Read the model definition and answer for the solid it produces. Units are mm, in the model's axes. Face numbers are marked on the shaded views. A direction names the side the tool comes from. Give positions to 0.01 mm unless a question says otherwise; leave off trailing zeros. Loops run counter-clockwise (first coordinate to the right, second up) from the corner with the lowest first, then second, coordinate; pieces in that order, holes last. Notation, with made-up numbers: (-5, 7.25) - (32, 7.25) arc R36 ccw to (32, 43.25) - close; hole circle Ø4 at (-3, 59). An arc over 180 degrees is marked (long way). Use a Markdown table: item, result. Add a question column.
Item 1: A cutting plane is placed at C-C (x = 11.5). Determine the outline of the cut face in (y, z), plus the area to 3 significant figures.
Item 2: Consider probe 1 along Y at (x, z) = (22.4, -2.5); probe 2 along X at (y, z) = (0.3, -2); probe 3 along Z at (x, y) = (10, 1.2). Determine where each line is inside the solid, lowest interval first. Write a range as [from, to].
Item 3: Which of the six approach directions +Z, -Z, +X, -X, +Y, -Y give full straight-line access (tool end or side, diameter ignored) to the marked faces 1 and 2?
Item 4: A cutting plane is placed at A-A (z = -5.25). Determine the outline of the cut face in (x, y), plus the area to 3 significant figures.
Item 5: For a pull along X with two mould halves and no side action, classify the marked faces 3, 4 and 5 as +X half, -X half, draft (parallel to the pull), parting line (faces both ways), or undercut.
Item 6: A cutting plane is placed at D-D (z = -2.5). Determine the outline of the cut face in (x, y), plus the area to 3 significant figures.
Item 7: A cutting plane is placed at B-B (y = 2.5). Determine the outline of the cut face in (x, z).
Item 8: Each of these flat-tipped pins is pushed along its axis until it touches: P1, Ø1.5, axis at y = 2.5, z = -11.5, coming from the +X side; P2, Ø2, axis at y = 3, z = -10, coming from the +X side. Where does it stop, or does it pass through?
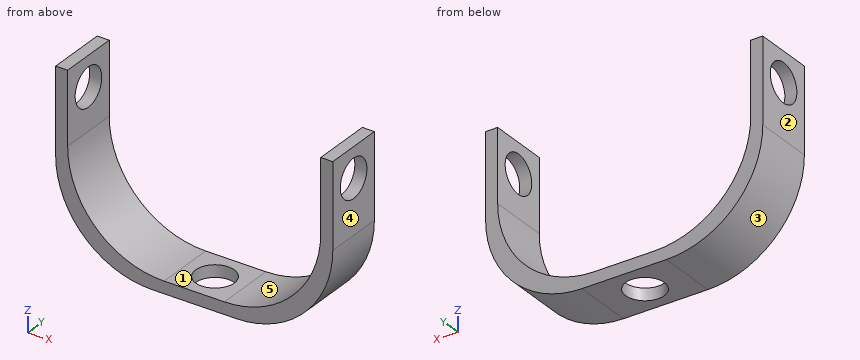
from build123d import *

# Parameters (mm, degrees)
BOSS_EXTRUDE1_DEPTH = 5
SKETCH2_R           = 1.6
CUT_EXTRUDE1_DEPTH  = 5
SKETCH3_R           = 1.6
CUT_EXTRUDE2_DEPTH  = 27
FILLET1_R           = 8


with BuildPart() as part:
    # Sketch1 → Boss-Extrude1 (new body)
    with BuildSketch(Plane(origin=(0, 0, 0), x_dir=(1, 0, 0), z_dir=(0, 1, 0))):
        Polygon((0, 0), (1, 0), (1, 14), (22, 14), (22, 0), (23, 0), (23, 15), (0, 15), align=None)
    extrude(amount=BOSS_EXTRUDE1_DEPTH)

    # Sketch2 → Cut-Extrude1 (cut)
    with BuildSketch(Plane(origin=(0, 0, -15), x_dir=(-1, 0, 0), z_dir=(0, 0, -1))):
        with Locations((-11.5, 2.5)):
            Circle(SKETCH2_R)
    extrude(amount=-CUT_EXTRUDE1_DEPTH, mode=Mode.SUBTRACT)

    # Sketch3 → Cut-Extrude2 (cut)
    with BuildSketch(Plane(origin=(23, 0, 0), x_dir=(0, 0, -1), z_dir=(1, 0, 0))):
        with Locations((2.5, 2.5)):
            Circle(SKETCH3_R)
    extrude(amount=-CUT_EXTRUDE2_DEPTH, mode=Mode.SUBTRACT)

    # Fillet1
    fillet1_edges = [part.edges().sort_by_distance(p)[0] for p in [
        (0, 2.5, -15),
        (23, 2.5, -15),
        (22, 2.5, -14),
        (1, 2.5, -14),
    ]]
    fillet(fillet1_edges, radius=FILLET1_R)


solid = part.part
Geometry says:
| question | item | result |
|---|---|---|
| 1 | outline | (0, -15) - (0.9, -15) - (0.9, -14) - (0, -14) - close; (4.1, -15) - (5, -15) - (5, -14) - (4.1, -14) - close |
| 1 | area | 1.80 mm² |
| 2 | probe 1 | [0, 0.9], [4.1, 5] |
| 2 | probe 2 | [0, 1], [22, 23] |
| 2 | probe 3 | [-15, -14] |
| 3 | face 1 | +Z, +Y, -Y |
| 3 | face 2 | +Z, -Z, -X, +Y, -Y |
| 4 | outline | (0, 0) - (1, 0) - (1, 5) - (0, 5) - close; (22, 0) - (23, 0) - (23, 5) - (22, 5) - close |
| 4 | area | 10.0 mm² |
| 5 | face 3 | -X half |
| 5 | face 4 | +X half |
| 5 | face 5 | undercut |
| 6 | outline | (0, 0) - (1, 0) - (1, 0.9) - (0, 0.9) - close; (0, 4.1) - (1, 4.1) - (1, 5) - (0, 5) - close; (22, 0) - (23, 0) - (23, 0.9) - (22, 0.9) - close; (22, 4.1) - (23, 4.1) - (23, 5) - (22, 5) - close |
| 6 | area | 3.60 mm² |
| 7 | outline | (0, -7) arc R8 ccw to (8, -15) - (9.9, -15) - (9.9, -14) - (9, -14) arc R8 cw to (1, -6) - (1, -4.1) - (0, -4.1) - close; (0, -0.9) - (1, -0.9) - (1, 0) - (0, 0) - close; (13.1, -15) - (15, -15) arc R8 ccw to (23, -7) - (23, -4.1) - (22, -4.1) - (22, -6) arc R8 cw to (14, -14) - (13.1, -14) - close; (22, -0.9) - (23, -0.9) - (23, 0) - (22, 0) - close |
| 8 | P1 | x = 22.07 |
| 8 | P2 | x = 22.75 |
